Autodesk Fusion 360 part; units mm, degrees
sketch "Boceto1" plane through (0, 0, 0) normal (0, 0, 1) x (1, 0, 0)
  line L0 (-38.0232, 20.8447) -> (47.9768, 20.8447)
  line L1 (47.9768, 20.8447) -> (47.9768, -12.6553)
  line L2 (47.9768, -12.6553) -> (-38.0232, -12.6553)
  line L3 (-38.0232, -12.6553) -> (-38.0232, 20.8447)
  line L4 (-41.0232, 23.8447) -> (50.9768, 23.8447)
  line L5 (50.9768, -15.6553) -> (-41.0232, -15.6553)
  line L6 (-38.0232, 20.8447) -> (-41.0232, 20.8447)
  line L7 (-41.0232, 20.8447) -> (50.9768, 20.8447)
  line L8 (-38.0232, -12.6553) -> (-41.0232, -12.6553)
  line L9 (-41.0232, -15.6553) -> (-41.0232, -12.6553)
  line L10 (-41.0232, 20.8447) -> (-41.0232, 23.8447)
  line L11 (47.9768, -12.6553) -> (50.9768, -12.6553)
  line L12 (50.9768, 23.8447) -> (50.9768, 20.8447)
  line L13 (50.9768, -12.6553) -> (50.9768, -15.6553)
  dimension "d1" = 86
  dimension "d2" = 33.5
  dimension "d3" = 3
  dimension "d4" = 3
  dimension "d5" = 3
  dimension "d6" = 3
extrude "Extruir1" add sketch "Boceto1" along normal blind 51 contours L0 L4 L6 L7 L10 L12 | L2 L5 L8 L9 L11 L13 makes body 1 at (20.3102, 20.8447, 17) makes body 2 at (20.3102, -12.6553, 17)
sketch "Boceto2" plane through (0, 0, 51) normal (0, 0, 1) x (-1, 0, 0)
  line L0 (41.0232, -20.8447) -> (-50.9768, -20.8447)
  line L1 (-50.9768, -20.8447) -> (-50.9768, -23.8447)
  line L2 (-50.9768, -23.8447) -> (41.0232, -23.8447)
  line L3 (41.0232, -23.8447) -> (41.0232, -20.8447)
  line L4 (41.0232, -23.8447) -> (-50.9768, -23.8447)
  line L5 (-50.9768, -23.8447) -> (-50.9768, 15.6553)
  line L6 (-50.9768, 15.6553) -> (41.0232, 15.6553)
  line L7 (41.0232, 15.6553) -> (41.0232, -23.8447)
  dimension "d9" = 39.5
  dimension "d12" = 92
extrude "Extruir2" add sketch "Boceto2" along normal blind 3 bodies 1 2
sketch "Boceto3" plane through (0, 0, 51) normal (0, 0, -1) x (1, 0, 0)
  line L0 (-41.0232, -20.8447) -> (50.9768, -20.8447)
  line L1 (50.9768, -20.8447) -> (50.9768, 12.6553)
  line L2 (50.9768, 12.6553) -> (-41.0232, 12.6553)
  line L3 (-41.0232, 12.6553) -> (-41.0232, -20.8447)
  line L4 (50.9768, 12.6553) -> (47.9768, 12.6553)
  line L5 (47.9768, 12.6553) -> (47.9768, 5.6553)
  line L6 (47.9768, 5.6553) -> (50.9768, 5.6553)
  line L7 (50.9768, 5.6553) -> (50.9768, 12.6553)
  line L8 (50.9768, -20.8447) -> (47.9768, -20.8447)
  line L9 (47.9768, -20.8447) -> (47.9768, -13.8447)
  line L10 (47.9768, -13.8447) -> (50.9768, -13.8447)
  line L11 (50.9768, -13.8447) -> (50.9768, -20.8447)
  dimension "d13" = 3
  dimension "d14" = 3
  dimension "d16" = 7
  dimension "d17" = 7
extrude "Extruir3" add sketch "Boceto3" along normal blind 51 contours L0 L1 L8 L9 L10 L11 | L1 L2 L4 L5 L6 L7 bodies 1
extrude "Extruir4" cut 1 faces at (50.9768, -12.322, 35) along direction (-1, 0, 0) blind 80 on bodies 1 bodies 1
extrude "Extruir5" add 2 faces at (-37.0232, -14.6553, 0) (-37.0232, 22.8447, 0) along direction (0, 0, -1) blind 0.75 on bodies 1 bodies 1
sketch "Boceto4" plane through (0, 0, -0.75) normal (0, 0, -1) x (1, 0, 0)
  line L0 (-29.0232, -23.8447) -> (-29.0232, -20.8447)
  line L1 (-29.0232, -20.8447) -> (-41.0232, -20.8447)
  line L2 (-41.0232, -20.8447) -> (-41.0232, -23.8447)
  line L3 (-41.0232, -23.8447) -> (-29.0232, -23.8447)
  line L4 (-35.0232, -23.8447) -> (-35.0232, -27.8447) construction
  dimension "d24" = 4
sketch "Boceto5" plane through (-41.0232, 0, 0) normal (-1, 0, 0) x (0, -1, 0)
  line L0 (-20.8447, -0.75) -> (-20.8447, 51)
  line L1 (-20.8447, 51) -> (12.6553, 51)
  line L2 (12.6553, 51) -> (12.6553, -0.75)
  line L3 (12.6553, -0.75) -> (15.6553, -0.75)
  line L4 (15.6553, -0.75) -> (15.6553, 54)
  line L5 (15.6553, 54) -> (-23.8447, 54)
  line L6 (-23.8447, 54) -> (-23.8447, -0.75)
  line L7 (-23.8447, -0.75) -> (-20.8447, -0.75)
  line L8 (15.6553, -0.75) -> (15.6553, 51) construction
  line L9 (12.6553, -0.75) -> (-20.8447, -0.75) construction
  line L10 (-4.0947, -0.75) -> (-4.0947, 51) construction
  line L11 (-4.0947, 25.125) -> (-4.0947, 51) construction
  line L12 (-4.0947, 38.0625) -> (-23.8447, 38.0625) construction
  line L13 (-4.0947, 38.0625) -> (12.6553, 38.0625) construction
  line L14 (12.6553, 38.0625) -> (19.6553, 38.0625) construction
  line L15 (-23.8447, 38.0625) -> (-27.8447, 38.0625) construction
  circle A0 centre (-27.8447, 38.0625) radius 4
  line L16 (-27.8447, 42.0625) -> (-23.8447, 42.0625)
  line L17 (-27.8447, 34.0625) -> (-23.8447, 34.0625)
  circle A1 centre (-27.8447, 38.0625) radius 1.5
  line L18 (19.6553, 42.0625) -> (15.6553, 42.0625)
  circle A2 centre (19.6553, 38.0625) radius 4
  circle A3 centre (19.6553, 38.0625) radius 1.5
  line L19 (19.6553, 34.0625) -> (15.6553, 34.0625)
  dimension "d25" = 7
  dimension "d26" = 4
  dimension "d27" = 3
extrude "Extruir6" add sketch "Boceto5" against normal blind 10 contours L6 A0 L17 | L6 A0 L16 | A0 | L4 A2 L19 | L4 L18 A2 | A2 bodies 1
equation "d12 = 86 mm + 6 mm"
equation "d25 = 3 mm + 4 mm"
Model file for the job. Use its own axes, mm. A direction names the side the tool comes from. Coordinates: 2 decimals unless noted, no trailing zeros. Write each loop counter-clockwise with the first axis right and the second up, starting at its lowest first coordinate (ties: lowest second). Pieces come first, ordered by that corner, then holes. Notation, with made-up numbers: (31.5, 59) - (44.5, 59) arc R10 cw to (44.5, 69) - close; hole circle Ø9 at (10, 87). An arc over 180 degrees is marked (long way). Write each question's results on one line, items separated by ' | '. Start each with the question number.
1) Cut at C-C (y = -17). Write the cut outline in (x, z).
2) Probe line 1 along Y through (x, z) = (-37.75, 28); line 2 along Y through (x, z) = (-39.75, 38.5); line 3 along Z through (x, y) = (-33.25, 2.5). List the from-to ranges inside material, lowest first. Write a range as from..to.
3) 3-axis set-ups, long thin cutter, end or side, ignore diameter. For faces 1 (the face through (-35, 20.845, 25)), 2 (the face through (-36, 26, 42.062)), 3 (the face through (-31.023, 26, 38)), 4 (the face through (-36, 26, 34.062)), 5 (the face through (-36, -18, 42.062)): which of +Z, -Z, +X, -X, +Y, -Y reach the whole face in a straight line?
4) Flat gauge pins, fed straight in: P1, Ø3.5, axis at y = -19.66, z = 38.06, coming from the +X side; P2, Ø1.5, axis at x = -32, y = -18, coming from the -Z side; P3, Ø2, axis at x = -35, y = 1.5, coming from the -Z side. Where does each tip first touch, or does it go through?
5) Mould opens along Z. For faces 6 (the face through (-36.093, 31.844, 38.15)), 7 (the face through (-36.09, -21.04, 37.49)), 8 (the face through (-35, 23.845, 26)), 9 (the face through (-36.093, 27.153, 36.732)) say: pulls with the +Z half, pulls with the -Z half, needs draft (parallel to the pull), parting line crosses it, or undercut.
6) Cut at A-A (z = 43.5). Write the cut outline in (x, y), then the cut area to 3 significant figures.
7) Cut at B-B (x = -39.75). Write the cut outline in (y, z).
Returned:
1) outline: (-41.02, 34.06) - (-31.02, 34.06) - (-31.02, 42.06) - (-41.02, 42.06) - close
2) line 1: -15.66..-12.66, 20.84..23.84 | line 2: -23.63..-21.09, -18.22..-12.66, 20.84..26.41, 29.28..31.82 | line 3: 51..54
3) face 1: -Z, +X, -X | face 2: +Z, +X, -X, +Y | face 3: +Z, -Z, +X, +Y | face 4: -Z, +X, -X, +Y | face 5: +Z, +X, -X, -Y
4) P1: x = -31.02 | P2: z = 34.06 | P3: z = 51
5) face 6: parting line crosses it | face 7: undercut | face 8: needs draft | face 9: undercut
6) outline: (-41.02, -15.66) - (-29.02, -15.66) - (-29.02, -12.66) - (-41.02, -12.66) - close; (-41.02, 20.84) - (-29.02, 20.84) - (-29.02, 23.84) - (-41.02, 23.84) - close | area: 72.0 mm^2
7) outline: (-19.66, 34.06) - (-15.66, 34.06) - (-15.66, -0.75) - (-12.66, -0.75) - (-12.66, 51) - (20.84, 51) - (20.84, -0.75) - (23.84, -0.75) - (23.84, 34.06) - (27.84, 34.06) arc R4 ccw to (27.84, 42.06) - (23.84, 42.06) - (23.84, 54) - (-15.66, 54) - (-15.66, 42.06) - (-19.66, 42.06) arc R4 ccw to start; hole circle Ø3 at (-19.66, 38.06); hole circle Ø3 at (27.84, 38.06)
